Input: part model. Units: mm. Frame: model coordinates. Face numbers are marked on the shaded views. Give positions to 0.01 mm unless a question says otherwise; leave off trailing zeros. Write each loop counter-clockwise with the first axis right and the second up, starting at its lowest first coordinate (ties: lowest second). Pieces come first, ordered by that corner, then holes. Notation, with made-up numbers: (13.25, 61) - (55.25, 61) arc R36 cw to (55.25, 97) - close; hole circle Ø9 at (45, 18.25). An arc over 180 degrees is marked (long way). Answer as a JSON object with one key per item and string values. Group by question number.
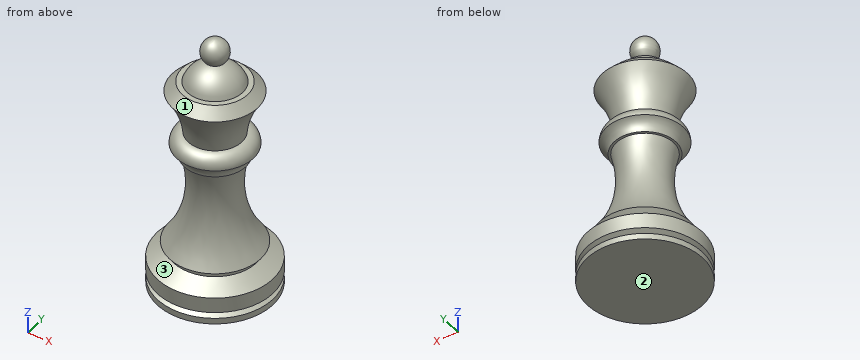
from build123d import *


# Not quite as in the source:
# - a feature names something its author has since deleted; it is built from what else it names


with BuildPart() as f1:
    # F0 (on Front) → F1 (revolve)
    with BuildSketch(Plane.XZ):
        with BuildLine():
            Line((0, 83.9221530378), (0, 52.0721530382))
            Line((0, 52.0721530382), (8.7499442067, 52.0721530382))
            Line((8.7499442067, 52.0721530382), (8.8241037769, 52.0721530382))
            ThreePointArc((8.8241037769, 52.0721530382), (10.4255958993, 59.4368383526), (13.9999442067, 66.0721530382))
            Line((13.9999442067, 66.0721530382), (10.7499442067, 69.3221530382))
            Line((10.7499442067, 69.3221530382), (9.08619756, 69.3221530382))
            ThreePointArc((9.08619756, 69.3221530382), (5.9884215444, 73.6392290372), (1.0750279815, 75.6620797781))
            ThreePointArc((1.0750279815, 75.6620797781), (4.1648192152, 80.2642011572), (0, 83.9221530378))
        make_face()
        with BuildLine():
            Line((0, 52.0721530382), (0, 48.041174956))
            Line((0, 48.041174956), (12.6061004532, 48.041174956))
            ThreePointArc((12.6061004532, 48.041174956), (11.5216028199, 50.8133495764), (8.8241037769, 52.0721530382))
            Line((8.8241037769, 52.0721530382), (8.7499442067, 52.0721530382))
            Line((8.7499442067, 52.0721530382), (0, 52.0721530382))
        make_face()
        with BuildLine():
            Line((0, 48.041174956), (0, 44.0721530382))
            Line((0, 44.0721530382), (9.4, 44.0721530382))
            Line((9.4, 44.0721530382), (10.13, 44.0721530382))
            ThreePointArc((10.13, 44.0721530382), (10.8184777766, 46.3995183881), (12.6061004532, 48.041174956))
            Line((12.6061004532, 48.041174956), (0, 48.041174956))
        make_face()
        Polygon((19, 0), (19, 1.9367265577), (17.2679491924, 2.9367265577), (19, 3.9367265577), (19, 8.9367265577), (13.5, 12.1121530382), (0, 12.1121530382), (0, 0), align=None)
        with BuildLine():
            Line((0, 44.0721530382), (0, 12.1121530382))
            Line((0, 12.1121530382), (13.5, 12.1121530382))
            Line((13.5, 12.1121530382), (13.5, 13.1121530382))
            Line((13.5, 13.1121530382), (15, 14.2461276344))
            ThreePointArc((15, 14.2461276344), (8.6430304158, 28.4912997708), (9.4, 44.0721530382))
            Line((9.4, 44.0721530382), (0, 44.0721530382))
        make_face()
    revolve(axis=Axis((0, 0, 41.9610765189), (0, 0, -1)))


solid = f1.part
1) Cut plane B-B on z = 20.5. Return the cut outline in (x, y), and give its area (3 significant figures).
2) Pin query (flat end, axial travel): P1, Ø2, axis at y = -2, z = 46, coming from the +X side; P2, Ø4, axis at y = -7.5, z = 73.5, coming from the -X side; P3, Ø6.5, axis at x = 3.5, y = 3.5, coming from the +Z side. Return the tip coordinate at first contact, or that it passes through.
3) Mould query, pull axis Z, two halves, no side actions, for the marked faces 1, 2 and 3. Classes: +Z half, -Z half, draft (parallel to the pull), parting line (faces both ways), or undercut.
4) Cut plane A-A on z = 41. Return the cut outline in (x, y), and give its area (3 significant figures).
5) Line query: line 1 along Z through (x, y) = (-12, -13.5); line 2 along Z through (x, y) = (9, -16); line 3 along Y through (x, z) = (-5.5, 62). Output: solid intervals per line, ascending. Write a range as from..to.
Filled in:
{
 "1": {"outline": "circle Ø22.42 at (0, 0)", "area": "395 mm²"},
 "2": {"P1": "stops at x = 11.1", "P2": "stops at x = -4.46", "P3": "stops at z = 83.56"},
 "3": {"face 1": "+Z half", "face 2": "-Z half", "face 3": "undercut"},
 "4": {"outline": "circle Ø17.32 at (0, 0)", "area": "236 mm²"},
 "5": {"line 1": "z = 0..2.48, 3.4..9.48", "line 2": "z = 0..2.31, 3.57..9.31", "line 3": "y = -10.13..10.13"}
}
